Geometry check sheet. Reference: the model listing, model coordinates, mm. A direction names the side the tool comes from. Coordinates: 2 decimals unless noted, no trailing zeros. Write each loop counter-clockwise with the first axis right and the second up, starting at its lowest first coordinate (ties: lowest second). Pieces come first, ordered by that corner, then holes. Notation, with made-up numbers: (-37.5, 62) -> (-33.5, 62) arc R33 cw to (-33.5, 98) -> close; hole circle Ø9 at (1.25, 22). An arc over 180 degrees is marked (long way). One line per question, with ' | ' between items.
```python
from build123d import *

# Parameters (mm, degrees)
F0_R     = 1.5
F0_R_2   = 12.5
F1_DEPTH = 6


with BuildPart() as f1:
    # F0 (on Front) → F1 (new body)
    with BuildSketch(Plane.XZ):
        with BuildLine():
            Line((-13.5, -27.5), (13.5, -27.5))
            ThreePointArc((13.5, -27.5), (14.56066, -27.06066), (15, -26))
            Line((15, -26), (15, 26))
            ThreePointArc((15, 26), (14.56066, 27.06066), (13.5, 27.5))
            Line((13.5, 27.5), (-13.5, 27.5))
            ThreePointArc((-13.5, 27.5), (-14.56066, 27.06066), (-15, 26))
            Line((-15, 26), (-15, -26))
            ThreePointArc((-15, -26), (-14.56066, -27.06066), (-13.5, -27.5))
        make_face()
        with Locations((-12.5, -25)):
            Circle(F0_R, mode=Mode.SUBTRACT)
        with Locations((12.5, -25)):
            Circle(F0_R, mode=Mode.SUBTRACT)
        with Locations((0, -12.5)):
            Circle(F0_R_2, mode=Mode.SUBTRACT)
        with Locations((-12.5, 0)):
            Circle(F0_R, mode=Mode.SUBTRACT)
        with BuildLine():
            Line((-9.295934, 22.325195), (-9.295934, 8.433623))
            ThreePointArc((-9.295934, 8.433623), (-10.045934, 7.683623), (-10.795934, 8.433623))
            Line((-10.795934, 8.433623), (-10.795934, 22.325195))
            ThreePointArc((-10.795934, 22.325195), (-10.045934, 23.075195), (-9.295934, 22.325195))
        make_face(mode=Mode.SUBTRACT)
        with Locations((12.5, 0)):
            Circle(F0_R, mode=Mode.SUBTRACT)
        with BuildLine():
            Line((10.795934, 22.325195), (10.795934, 8.433623))
            ThreePointArc((10.795934, 8.433623), (10.045934, 7.683623), (9.295934, 8.433623))
            Line((9.295934, 8.433623), (9.295934, 22.325195))
            ThreePointArc((9.295934, 22.325195), (10.045934, 23.075195), (10.795934, 22.325195))
        make_face(mode=Mode.SUBTRACT)
    extrude(amount=F1_DEPTH)


solid = f1.part
```
(1) Cross-section at A-A (z = -12.5). Record the cut outline in (x, y).
Answers below:
outline: (-15, -6) -> (-12.5, -6) -> (-12.5, 0) -> (-15, 0) -> close; (12.5, -6) -> (15, -6) -> (15, 0) -> (12.5, 0) -> close
(2) Cross-section at B-B (y = -4.45). Record the cut outline in (x, z).
Answers below:
outline: (-15, -26) arc R1.5 ccw to (-13.5, -27.5) -> (13.5, -27.5) arc R1.5 ccw to (15, -26) -> (15, 26) arc R1.5 ccw to (13.5, 27.5) -> (-13.5, 27.5) arc R1.5 ccw to (-15, 26) -> close; hole circle Ø3 at (-12.5, -25); hole circle Ø3 at (-12.5, 0); hole circle Ø25 at (0, -12.5); hole (-10.8, 8.43) arc R0.75 ccw to (-9.3, 8.43) -> (-9.3, 22.33) arc R0.75 ccw to (-10.8, 22.33) -> close; hole (9.3, 8.43) arc R0.75 ccw to (10.8, 8.43) -> (10.8, 22.33) arc R0.75 ccw to (9.3, 22.33) -> close; hole circle Ø3 at (12.5, -25); hole circle Ø3 at (12.5, 0)
(3) Material ranges on line 1 (X direction, y = -5.65, z = 20); line 2 (Z direction, x = 0, y = -1.5); line 3 (Z direction, x = 10.5, y = -3.7), recorded low to high.
Answers below:
line 1: x = -15 to -10.8, -9.3 to 9.3, 10.8 to 15 | line 2: z = -27.5 to -25, 0 to 27.5 | line 3: z = -27.5 to -19.28, -5.72 to 7.84, 22.92 to 27.5
(4) Cross-section at D-D (z = 10). Record the cut outline in (x, y), plus the area to 3 significant figures.
Answers below:
outline: (-15, -6) -> (-10.8, -6) -> (-10.8, 0) -> (-15, 0) -> close; (-9.3, -6) -> (9.3, -6) -> (9.3, 0) -> (-9.3, 0) -> close; (10.8, -6) -> (15, -6) -> (15, 0) -> (10.8, 0) -> close | area: 162 mm²
(5) Tool access check on faces 4 (the face through (14.57, -2.96, 27.05)), 5 (the face through (-10.062, -2.958, 23.075)). Record the directions out of +Z, -Z, +X, -X, +Y, -Y that give a thin tool (end or side, any length) a straight path to the whole face; none if there is none.
Answers below:
face 4: +Z, +X, +Y, -Y | face 5: +Y, -Y
(6) Draft check along Z on faces 1 (the face through (15, -3, 0)), 2 (the face through (-9.296, -3, 15)), 3 (the face through (0, -3, 27.5)). Enter one of: pulls with the +Z half, pulls with the -Z half, needs draft (parallel to the pull), parting line crosses it, or undercut.
Answers below:
face 1: needs draft | face 2: undercut | face 3: pulls with the +Z half
(7) Cross-section at C-C (x = 0). Record the cut outline in (y, z), plus the area to 3 significant figures.
Answers below:
outline: (-6, -27.5) -> (0, -27.5) -> (0, -25) -> (-6, -25) -> close; (-6, 0) -> (0, 0) -> (0, 27.5) -> (-6, 27.5) -> close | area: 180 mm²
